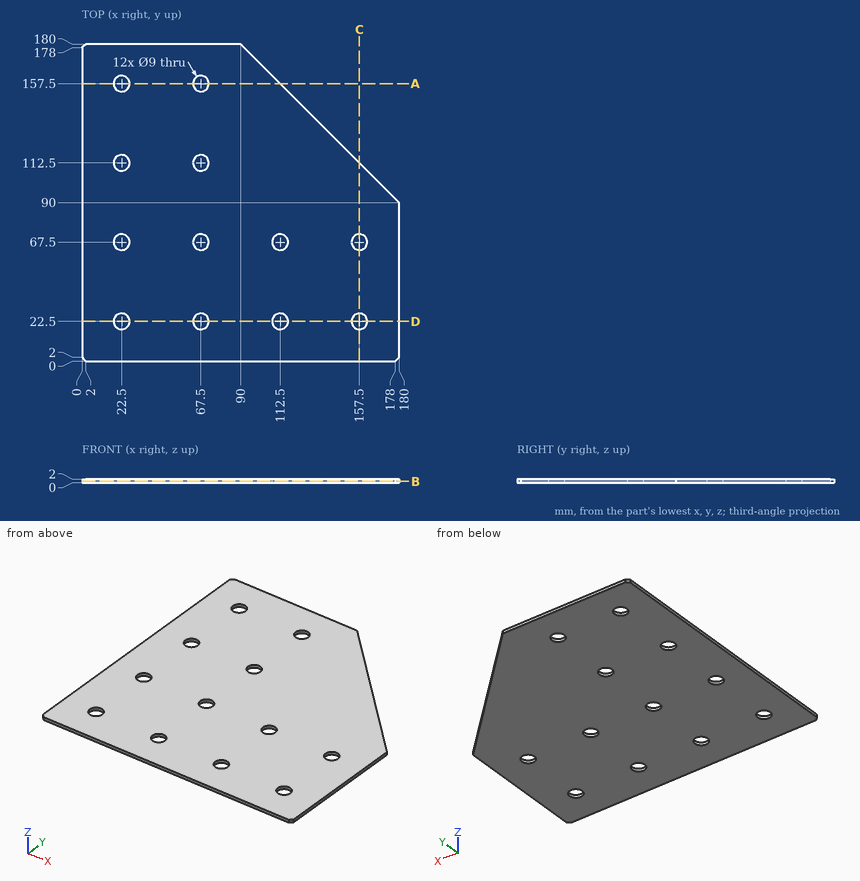
Study the drawing (mm; zero at the part's minimum x, y, z) and answer. Coordinates: 2 decimals unless noted, no trailing zeros. Write each loop counter-clockwise with the first axis right and the second up, starting at its lowest first coordinate (ties: lowest second). Pieces come first, ordered by that corner, then holes. Notation, with made-up numbers: (-26, 85) - (7, 85) arc R12 ccw to (7, 99) - close; hole circle Ø4 at (55.25, -14.75). An arc over 180 degrees is marked (long way). Answer as a JSON object with one key per item and string values.
Q1. Find section D-D (y = 22.5). Write down the section's boundary in (x, z), plus the area to 3 significant figures.
Results list:
{"outline": "(0, 0) - (18, 0) - (18, 2) - (0, 2) - close; (27, 0) - (63, 0) - (63, 2) - (27, 2) - close; (72, 0) - (108, 0) - (108, 2) - (72, 2) - close; (117, 0) - (153, 0) - (153, 2) - (117, 2) - close; (162, 0) - (180, 0) - (180, 2) - (162, 2) - close", "area": "288 mm^2"}
Q2. Find section A-A (y = 157.5). Write down the section's boundary in (x, z).
Results list:
{"outline": "(0, 0) - (18, 0) - (18, 2) - (0, 2) - close; (27, 0) - (63, 0) - (63, 2) - (27, 2) - close; (72, 0) - (112.5, 0) - (112.5, 2) - (72, 2) - close"}
Q3. Given pin 1 Ø8 at (x, y) = (22.5, 112.5) entering from +Z, flat-ended and moving along its own axis, determine where the tip first touches the part or whether it passes through.
Results list:
{"pin 1": "passes through"}
Q4. Find section B-B (z = 0.6). State how many separate pieces and enclosed holes the cut face has, plus the area to 3 significant figures.
Results list:
{"separate pieces": "1", "enclosed holes": "12", "area": "27,600 mm^2"}
Q5. Consider L1, parallel to Y at x = 22, z = 1.4; L2, parallel to X at y = 67.5, z = 1.25; L3, parallel to X at y = 158, z = 0.65. Determine where each line is inside the solid, lowest interval first. Write a range as from..to.
Results list:
{"L1": "y = 0..18.03, 26.97..63.03, 71.97..108.03, 116.97..153.03, 161.97..180", "L2": "x = 0..18, 27..63, 72..108, 117..153, 162..180", "L3": "x = 0..18.03, 26.97..63.03, 71.97..112"}
